from build123d import *

# Parameters (mm, degrees)
SKETCH1_R           = 2.5
BOSS_EXTRUDE1_DEPTH = 10


with BuildPart() as part:
    # Sketch1 → Boss-Extrude1 (new body)
    with BuildSketch(Plane.XY):
        with BuildLine():
            Line((-7.5, 0), (-7.5, 50))
            ThreePointArc((-7.5, 50), (0, 57.5), (7.5, 50))
            ThreePointArc((7.5, 50), (18.481305966, 21.383175369), (45.787292818, 7.458563536))
            ThreePointArc((45.787292818, 7.458563536), (52.48963372, -0.394191248), (45, -7.5))
            Line((45, -7.5), (0, -7.5))
            ThreePointArc((0, -7.5), (-5.303300859, -5.303300859), (-7.5, 0))
        make_face()
        Circle(SKETCH1_R, mode=Mode.SUBTRACT)
        with Locations((45, 0)):
            Circle(SKETCH1_R, mode=Mode.SUBTRACT)
        with Locations((0, 50)):
            Circle(SKETCH1_R, mode=Mode.SUBTRACT)
    extrude(amount=BOSS_EXTRUDE1_DEPTH)


solid = part.part
Here's how the part is built. I have some questions about the finished solid (model axes, mm). Coordinates: 2 decimals unless noted, no trailing zeros. Order: outer loops, then holes, each group sorted by start corner. A loop starts at its lowest first (then second) coordinate and runs counter-clockwise, first axis right, second up. Notation, with made-up numbers: M 47.5,38 L 57.5,38 A11 cw 57.5,53 Z; hole C -21,17 d5. An arc over 180 degrees is marked long. Answer as CSV lines item,"result". Start each with the question number.
1. We'd pull the mould along Y, two halves only. Please class faces 1 (the cylindrical face through (-0.54, -2.44, 4.93)), 2 (the flat face through (23, -7.5, 5)), 3 (the flat face through (-7.5, 25, 5)), 4 (the cylindrical face through (-0.54, 47.56, 4.93)): released by +Y, released by -Y, zero draft, split by the parting line, or undercut.
2. I want a section at C-C, the plane y = 44.5. Write out the boundary of the cut face in (x, z).
3. I want a section at B-B, the plane y = 34. Write out the boundary of the cut face in (x, z).
4. I need wall thicknesses on line 1 (Y direction, x = 0, z = 4.5); line 2 (X direction, y = 48, z = 1); line 3 (Y direction, x = 46, z = 5). Which ranges of each line are inside material? Lowest first, please. Write a range as [from, to].
5. I want a section at A-A, the plane z = 1. Write out the boundary of the cut face in (x, y).
6. For pin 1 (4.5 mm diameter, centred on x = 0, y = 50, fed in from +Z); pin 2 (1.5 mm diameter, centred on y = 40.5, z = 8, fed in from +X); pin 3 (1 mm diameter, centred on y = 38.5, z = 3, fed in from +X), each with a flat end and sliding along its axis, tell me the tip position at first contact or that it passes through.
Recorded:
1,face 1,"undercut"
1,face 2,"released by -Y"
1,face 3,"zero draft"
1,face 4,"undercut"
2,outline,"M -7.5,0 L 7.86,0 L 7.86,10 L -7.5,10 Z"
3,outline,"M -7.5,0 L 10.6,0 L 10.6,10 L -7.5,10 Z"
4,line 1,"y = [-7.5, -2.5], [2.5, 47.5], [52.5, 57.5]"
4,line 2,"x = [-7.5, -1.5], [1.5, 7.55]"
4,line 3,"y = [-7.43, -2.29], [2.29, 7.43]"
5,outline,"M -7.5,0 A7.5 ccw 0,-7.5 L 45,-7.5 A7.5 ccw 45.79,7.46 A42.78 cw 7.5,50 A7.5 ccw -7.5,50 Z; hole C 0,0 d5; hole C 0,50 d5; hole C 45,0 d5"
6,pin 1,"passes through"
6,pin 2,"stops at x = 8.75"
6,pin 3,"stops at x = 9.22"
